Print and shaded views of the part. All mm, measured from the part's lowest x, y and z. Round coordinates to 2 decimals unless told otherwise and drop trailing zeros. Loops run counter-clockwise (first coordinate to the right, second up) from the corner with the lowest first, then second, coordinate; pieces in that order, holes last. Notation, with made-up numbers: (47, -9) - (96, -9) arc R16 ccw to (96, 16) - close; hole circle Ø8 at (50.25, -34.75). An arc over 180 degrees is marked (long way). Answer as a JSON object with one key per item and string values.
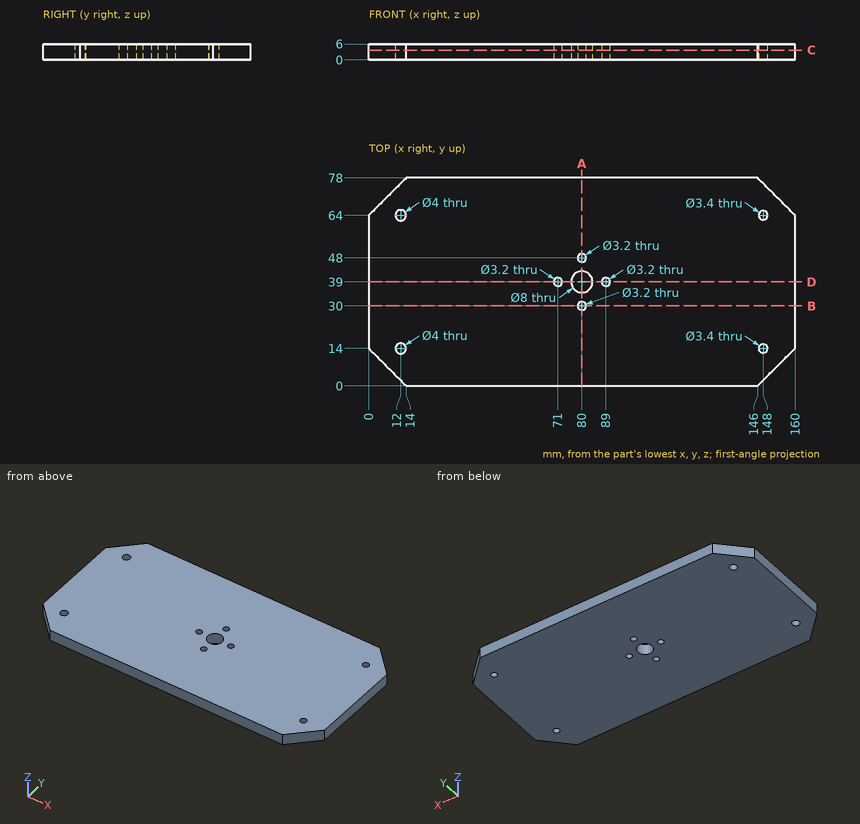
1) Slice it at A-A on x = 80. List the corners of the cut face in (y, z), then the cut area to 3 significant figures.
Values follow:
{"outline": "(0, 0) - (28.4, 0) - (28.4, 6) - (0, 6) - close; (31.6, 0) - (35, 0) - (35, 6) - (31.6, 6) - close; (43, 0) - (46.4, 0) - (46.4, 6) - (43, 6) - close; (49.6, 0) - (78, 0) - (78, 6) - (49.6, 6) - close", "area": "382 mm²"}
2) Slice it at B-B on y = 30. List the corners of the cut face in (x, z).
Values follow:
{"outline": "(0, 0) - (78.4, 0) - (78.4, 6) - (0, 6) - close; (81.6, 0) - (160, 0) - (160, 6) - (81.6, 6) - close"}
3) Slice it at D-D on y = 39. List the corners of the cut face in (x, z).
Values follow:
{"outline": "(0, 0) - (69.4, 0) - (69.4, 6) - (0, 6) - close; (72.6, 0) - (76, 0) - (76, 6) - (72.6, 6) - close; (84, 0) - (87.4, 0) - (87.4, 6) - (84, 6) - close; (90.6, 0) - (160, 0) - (160, 6) - (90.6, 6) - close"}
4) Probe probe 1 along X at (y, z) = (64, 3.25); probe 2 along Y at (x, z) = (80, 2.6); probe 3 along Y at (x, z) = (148, 1.55). List the from-to ranges inside material, lowest first.
Values follow:
{"probe 1": "0 to 10, 14 to 146.3, 149.7 to 160", "probe 2": "0 to 28.4, 31.6 to 35, 43 to 46.4, 49.6 to 78", "probe 3": "2 to 12.3, 15.7 to 62.3, 65.7 to 76"}
5) Slice it at C-C on z = 3.7. Count the separate pieces of the cut face and the enclosed holes in it, then the cut area to 3 significant figures.
Values follow:
{"separate pieces": "1", "enclosed holes": "9", "area": "12,000 mm²"}
